from build123d import *

# Parameters (mm, degrees)
F1_DEPTH      = 25.4
F3_DEPTH      = 5.08
F3_DEPTH_BACK = 2.54
F4_R          = 2.54
F6_DEPTH      = 3.048


with BuildPart() as f1:
    # F0 (on Top) → F1 (new body)
    with BuildSketch(Plane.XY):
        Polygon((6.35, -19.05), (31.75, -19.05), (31.75, -46.0375), (38.1, -46.0375), (38.1, -12.7), (0, -12.7), (0, -46.0375), (6.35, -46.0375), align=None)
    extrude(amount=F1_DEPTH)

    # F2 (on face) → F3 (join, two sides)
    with BuildSketch(Plane.XY.offset(25.4)) as f3_sk:
        Polygon((0, -46.0375), (0, -19.05), (-9.525, -19.05), (-6.35, -46.0375), align=None)
    extrude(amount=-F3_DEPTH)
    extrude(f3_sk.sketch, amount=F3_DEPTH_BACK)

    # F4
    f4_edges = [f1.edges().sort_by_distance(p)[0] for p in [
        (6.35, -19.05, 12.7),
        (31.75, -19.05, 12.7),
        (38.1, -12.7, 12.7),
        (0, -12.7, 12.7),
    ]]
    fillet(f4_edges, radius=F4_R)

    # F5 (on face) → F6 (cut)
    with BuildSketch(Plane(origin=(0, 0, 20.32), x_dir=(1, 0, 0), z_dir=(0, 0, -1))):
        Polygon((0, 46.0375), (-4.4318619133, 46.0375), (-7.6068619133, 19.05), (0, 19.05), align=None)
    extrude(amount=-F6_DEPTH, mode=Mode.SUBTRACT)


solid = f1.part
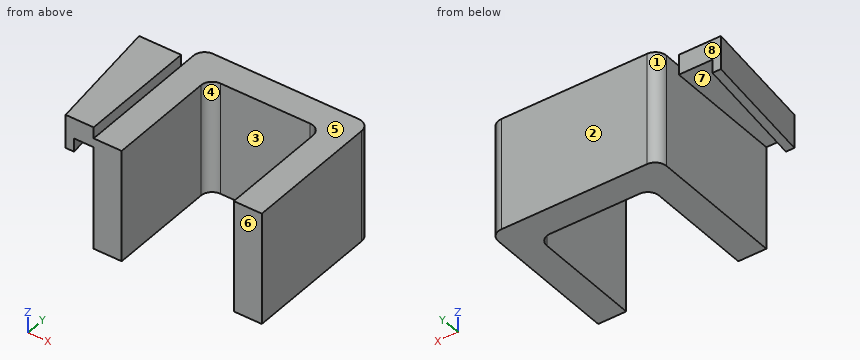
For this review, take the finished solid that the model builds, in its own axes (mm). Face numbers are marked on the shaded views. A direction names the side the tool comes from. Round coordinates to 2 decimals unless told otherwise and drop trailing zeros. Loops run counter-clockwise (first coordinate to the right, second up) from the corner with the lowest first, then second, coordinate; pieces in that order, holes last. Notation, with made-up numbers: (51.25, 21) - (93.25, 21) arc R32 ccw to (93.25, 57) - close; hole circle Ø3 at (58.25, 10.5). An arc over 180 degrees is marked (long way). Use one line per item in the form item = value.
1) We need section C-C on x = 24. Write out the cut boundary in (y, z).
Solutions:
outline = (-19.05, 0) - (-12.7, 0) - (-12.7, 25.4) - (-19.05, 25.4) - close
2) Clearance check with flat-ended pins moving along their axes: P1, Ø10, axis at y = -40.5, z = 16.5, coming from the -X side; P2, Ø12, axis at y = -29.5, z = 19, coming from the -X side; P3, Ø4, axis at x = -4, y = -27, coming from the -Z side. State where each tip first meets the part, or that it passes through.
Solutions:
P1 = -7.38
P2 = -8.98
P3 = 23.37
3) Mouldability with a two-part tool opening along X and no side actions: class the marked faces 1, 2 and 3 as pulls with the +X half, pulls with the -X half, needs draft (parallel to the pull), parting line crosses it, or undercut.
Solutions:
face_1 = pulls with the -X half
face_2 = needs draft
face_3 = undercut
4) Wall thickness on probe 1 along X at (y, z) = (-30, 4.5); probe 2 along Y at (x, z) = (21.5, 8): over which ranges is each line inside the solid? List them lowest first.
Solutions:
probe_1 = 0 to 6.35, 31.75 to 38.1
probe_2 = -19.05 to -12.7
5) Tool access review of the marked faces 4, 5, 6, 7 and 8: name each direction out of +Z, -Z, +X, -X, +Y, -Y from which nothing blocks a thin tool from reaching the whole face with its end or side.
Solutions:
face_4 = +Z, -Z, -Y
face_5 = +Z, +X, +Y, -Y
face_6 = +Z, -Z, +X, -X, -Y
face_7 = -Z, +Y
face_8 = +Z, -Z, -X, +Y
6) We need section A-A on y = -37. Write out the cut boundary in (x, z), then the cut area to 3 significant figures.
Solutions:
outline = (-7.41, 20.32) - (-5.5, 20.32) - (-5.5, 23.37) - (0, 23.37) - (0, 0) - (6.35, 0) - (6.35, 25.4) - (0, 25.4) - (0, 27.94) - (-7.41, 27.94) - close; (31.75, 0) - (38.1, 0) - (38.1, 25.4) - (31.75, 25.4) - close
area = 362 mm2
7) We need section B-B on z = 5. Write out the cut boundary in (x, y), then the cut area to 3 significant figures.
Solutions:
outline = (0, -46.04) - (6.35, -46.04) - (6.35, -21.59) arc R2.54 cw to (8.89, -19.05) - (29.21, -19.05) arc R2.54 cw to (31.75, -21.59) - (31.75, -46.04) - (38.1, -46.04) - (38.1, -15.24) arc R2.54 ccw to (35.56, -12.7) - (2.54, -12.7) arc R2.54 ccw to (0, -15.24) - close
area = 585 mm2
